from build123d import *

# Parameters (mm, degrees)
F0_W     = 363.556385
F0_H     = 250
F0_W_2   = 386.443615
F1_DEPTH = 50


with BuildPart() as f1:
    # F0 (on Front) → F1 (new body)
    with BuildSketch(Plane.XZ):
        Polygon((0, 150), (0, 500), (-576.39432, 0), (0, -500), (0, -150), (800, -150), (800, 150), align=None)
        Polygon((-455.829133, -71.490273), (-25, -71.490273), (-25, -420.501658), (-25, -445.218048), (-284.563661, -220.056511), align=None, mode=Mode.SUBTRACT)
        Polygon((-25, 445.218048), (-25, -41.858591), (-455.829133, -41.858591), (-489.988199, -41.858591), (-538.242307, 0), align=None, mode=Mode.SUBTRACT)
        with Locations((181.778192, 0)):
            Rectangle(F0_W, F0_H, mode=Mode.SUBTRACT)
        with Locations((581.778192, 0)):
            Rectangle(F0_W_2, F0_H, mode=Mode.SUBTRACT)
    extrude(amount=F1_DEPTH)


solid = f1.part
The listing builds one solid part. Answer for the finished solid, in the listing's coordinates (mm). A direction names the side the tool comes from. Give positions to 0.01 mm unless a question says otherwise; leave off trailing zeros. Write each loop counter-clockwise with the first axis right and the second up, starting at its lowest first coordinate (ties: lowest second). Pieces come first, ordered by that corner, then holes. Notation, with made-up numbers: (78.25, -5.75) -> (95.25, -5.75) arc R9 cw to (95.25, 8.25) -> close; hole circle Ø6 at (24, -16). An arc over 180 degrees is marked (long way). Use a Markdown table: item, result.
(1) Section D-D, the plane z = 66 is taken. Determine the outline of the cut face in (x, y).
Return value:
| item | result |
|---|---|
| outline | (-500.31, -50) -> (-462.16, -50) -> (-462.16, 0) -> (-500.31, 0) -> close; (-25, -50) -> (0, -50) -> (0, 0) -> (-25, 0) -> close; (363.56, -50) -> (388.56, -50) -> (388.56, 0) -> (363.56, 0) -> close; (775, -50) -> (800, -50) -> (800, 0) -> (775, 0) -> close |
(2) Section B-B, the plane z = 372.5 is taken. Determine the outline of the cut face in (x, y).
Return value:
| item | result |
|---|---|
| outline | (-146.98, -50) -> (-108.83, -50) -> (-108.83, 0) -> (-146.98, 0) -> close; (-25, -50) -> (0, -50) -> (0, 0) -> (-25, 0) -> close |
(3) Flat-ended cylindrical pins translate along their axes: P1, Ø25, axis at y = -27.5, z = 317, coming from the +X side; P2, Ø12, axis at x = 128.5, y = -17, coming from the +Z side; P3, Ø15, axis at y = -17.5, z = -175.5, coming from the -X side. Find the tip coordinate at first contact, or state that the pin passes through.
Return value:
| item | result |
|---|---|
| P1 | x = 0 |
| P2 | z = 150 |
| P3 | x = -382.73 |
(4) Section C-C, the plane y = -9 is taken. Determine the outline of the cut face in (x, z), then the cut area to 3 significant figures.
Return value:
| item | result |
|---|---|
| outline | (-576.39, 0) -> (0, -500) -> (0, -150) -> (800, -150) -> (800, 150) -> (0, 150) -> (0, 500) -> close; hole (-538.24, 0) -> (-489.99, -41.86) -> (-25, -41.86) -> (-25, 445.22) -> close; hole (-455.83, -71.49) -> (-25, -445.22) -> (-25, -71.49) -> close; hole (0, -125) -> (363.56, -125) -> (363.56, 125) -> (0, 125) -> close; hole (388.56, -125) -> (775, -125) -> (775, 125) -> (388.56, 125) -> close |
| area | 125,000 mm2 |
(5) For faces 5 (the flat face through (179, -25, 125)), 6 (the flat face through (800, -25, -2)), determine the directions among +Z, -Z, +X, -X, +Y, -Y from which every point of the face is accessible in a straight line to the end or side of a thin tool.
Return value:
| item | result |
|---|---|
| face 5 | +Y, -Y |
| face 6 | +Z, -Z, +X, +Y, -Y |
(6) Section A-A, the plane x = 255.5 is taken. Determine the outline of the cut face in (y, z), then the cut area to 3 significant figures.
Return value:
| item | result |
|---|---|
| outline | (-50, -150) -> (0, -150) -> (0, -125) -> (-50, -125) -> close; (-50, 125) -> (0, 125) -> (0, 150) -> (-50, 150) -> close |
| area | 2,500 mm2 |
(7) Find the intervals of material crossed by probe 1 along Z at (x, y) = (108, -16.5); probe 2 along Z at (x, y) = (-175.5, -11.5); probe 3 along X at (y, z) = (-9.5, 16), in increasing order. Write a range as from..to.
Return value:
| item | result |
|---|---|
| probe 1 | -150..-125, 125..150 |
| probe 2 | -347.76..-314.67, -71.49..-41.86, 314.67..347.76 |
| probe 3 | -557.95..-519.8, -25..0, 363.56..388.56, 775..800 |
(8) Determine the mould class of faces 1 (the flat face through (388.556, -25, -2)), 2 (the flat face through (394, -25, -150)), 3 (the flat face through (-284.16, -24.65, 253.5)), 4 (the flat face through (0, -25, 323)) for opening direction Z: released by +Z, released by -Z, zero draft, split by the parting line, or undercut.
Return value:
| item | result |
|---|---|
| face 1 | undercut |
| face 2 | released by -Z |
| face 3 | released by +Z |
| face 4 | zero draft |
